```python
from build123d import *

# Parameters (mm, degrees)
BLANKSKE_W          = 100
BLANKSKE_H          = 11
BLANK_DEPTH         = 12
TOOTHCUTSIM_DEPTH   = 102.316336294
TEETHCUTS_COUNT     = 33
TEETHCUTS_PITCH     = 3.14159265
SKETCH1_W           = 12
SKETCH1_H           = 5.53
CUT_EXTRUDE1_DEPTH  = 126
SKETCH2_W           = 12
SKETCH2_H           = 3.457737656
BOSS_EXTRUDE1_DEPTH = 5
SKETCH3_W           = 5
SKETCH3_H           = 12
BOSS_EXTRUDE2_DEPTH = 50
FILLET1_R           = 5
SKETCH4_W           = 10
SKETCH4_H           = 3.22
BOSS_EXTRUDE3_DEPTH = 10
FILLET2_R           = 3


with BuildPart() as part:
    # BlankSke → Blank (new body)
    with BuildSketch(Plane.XY):
        with Locations((50, 5.5)):
            Rectangle(BLANKSKE_W, BLANKSKE_H)
    extrude(amount=-BLANK_DEPTH)

    # TooCutSkeSim → ToothCutSim (cut, through all)
    with BuildSketch(Plane.XY):
        Polygon((0.44443537, 8.75), (-0.44443537, 8.75), (-1.272613241, 11.0254), (1.272613241, 11.0254), align=None)
    toothcutsim = extrude(amount=-TOOTHCUTSIM_DEPTH, mode=Mode.SUBTRACT)

    # TeethCuts: ToothCutSim ×33
    with Locations(*[(i * TEETHCUTS_PITCH, 0, 0) for i in range(1, TEETHCUTS_COUNT)]):
        add(toothcutsim, mode=Mode.SUBTRACT)

    # Sketch1 → Cut-Extrude1 (cut)
    with BuildSketch(Plane(origin=(100, 0, 0), x_dir=(0, 0, -1), z_dir=(1, 0, 0))):
        with Locations((6, 2.765)):
            Rectangle(SKETCH1_W, SKETCH1_H)
    extrude(amount=-CUT_EXTRUDE1_DEPTH, mode=Mode.SUBTRACT)

    # Sketch2 → Boss-Extrude1 (add)
    with BuildSketch(Plane(origin=(100, 0, 0), x_dir=(0, 0, -1), z_dir=(1, 0, 0))):
        with Locations((6, 7.258868828)):
            Rectangle(SKETCH2_W, SKETCH2_H)
    extrude(amount=BOSS_EXTRUDE1_DEPTH)

    # Sketch3 → Boss-Extrude2 (add)
    with BuildSketch(Plane.XZ.offset(-5.53)):
        with Locations((102.5, -6)):
            Rectangle(SKETCH3_W, SKETCH3_H)
    extrude(amount=BOSS_EXTRUDE2_DEPTH)

    # Fillet1
    fillet1_edges = [part.edges().sort_by_distance(p)[0] for p in [
        (100, 5.53, -6),
    ]]
    fillet(fillet1_edges, radius=FILLET1_R)

    # Sketch4 → Boss-Extrude3 (add)
    with BuildSketch(Plane(origin=(0, 0, -12), x_dir=(-1, 0, 0), z_dir=(0, 0, -1))):
        with Locations((-5, 7.14)):
            Rectangle(SKETCH4_W, SKETCH4_H)
    extrude(amount=BOSS_EXTRUDE3_DEPTH)

    # Fillet2
    # the kernel refuses this fillet: 3 mm, written as the material it adds along each edge
    with BuildSketch(Plane(origin=(10, 5.53, -12), x_dir=(1, 0, 0), z_dir=(0, 1, 0))) as fillet2_piece_1:
        with BuildLine():
            CenterArc((FILLET2_R, FILLET2_R), FILLET2_R, 180, 90)
            Line((0, FILLET2_R), (0, 0))
            Line((0, 0), (FILLET2_R, 0))
        make_face()
    extrude(amount=3.22)


solid = part.part
```
Design review of the part built by this model. Coordinates are the model's own, in mm. A direction names the side the tool comes from. Coordinates: 2 decimals unless noted, no trailing zeros. Order: outer loops, then holes, each group sorted by start corner. A loop starts at its lowest first (then second) coordinate and runs counter-clockwise, first axis right, second up. Notation, with made-up numbers: M 46,45.25 L 60,45.25 A18 cw 60,52.25 Z; hole C 83,14.25 d2. An arc over 180 degrees is marked long. Answer as a JSON object with one key per item and string values. Group by question number.
1) Add section A-A, the plane y = -17.5. Write out the cut boundary in (x, z), then the cut area to 3 significant figures.
2) Mouldability with a two-part tool opening along X and no side actions: class faces 4 (the flat face through (13.426, 9.891, -5.916)), 5 (the flat face through (48, 5.53, -6)), 6 (the flat face through (10, 7, -18)) as pulls with the +X half, pulls with the -X half, needs draft (parallel to the pull), parting line crosses it, or undercut.
3) Wall thickness on L1, parallel to X at y = -28, z = -4.5; L2, parallel to Y at x = 44, z = -11.75; L3, parallel to Z at x = 83, y = 8.5: over which ranges is each line inside the solid? List them lowest first.
4) For pin 1 (6 mm diameter, centred on x = 81.5, z = -3.5, fed in from -Y); pin 2 (12 mm diameter, centred on y = -36.5, z = -14, fed in from -X); pin 3 (5.5 mm diameter, centred on x = 101.5, z = -3.5, fed in from +Y); pin 4 (3 mm diameter, centred on y = 1.5, z = -3, fed in from -X), all flat-tipped, find the tip position at first contact; note any pin that passes through.
5) Add section B-B, the plane z = -17. Write out the cut boundary in (x, y).
6) Tool access review of faces 1 (the flat face through (99.64, 9.98, -5.92)), 2 (the flat face through (72, 6, -12)), 3 (the flat face through (54.267, 9.891, -5.916)): name each direction out of +Z, -Z, +X, -X, +Y, -Y from which nothing blocks a thin tool from reaching the whole face with its end or side.
Computed values:
{
 "1": {"outline": "M 100,-12 L 105,-12 L 105,0 L 100,0 Z", "area": "60.0 mm^2"},
 "2": {"face 4": "undercut", "face 5": "needs draft", "face 6": "pulls with the +X half"},
 "3": {"L1": "x = 100 to 105", "L2": "y = 5.53 to 8.75", "L3": "z = -12 to 0"},
 "4": {"pin 1": "stops at y = 5.53", "pin 2": "stops at x = 100", "pin 3": "stops at y = 11", "pin 4": "stops at x = 99.35"},
 "5": {"outline": "M 0,5.53 L 10,5.53 L 10,8.75 L 0,8.75 Z"},
 "6": {"face 1": "+Z, -Z, +X, +Y", "face 2": "-Z, +X, +Y, -Y", "face 3": "+Z, -Z, +Y"}
}
